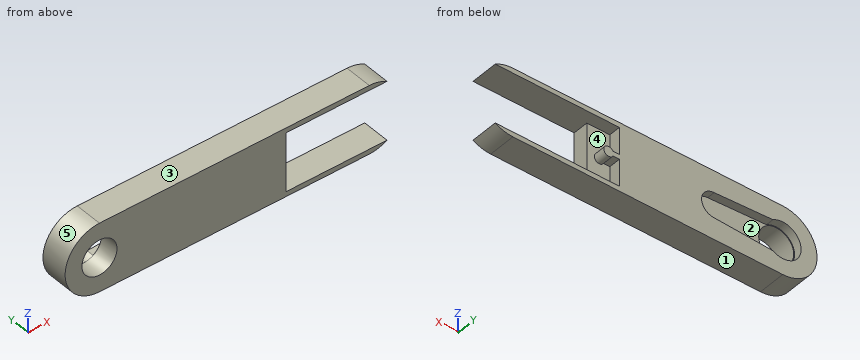
from build123d import *

# Parameters (mm, degrees)
BOSS_EXTRUDE1_DEPTH = 3.95
SKETCH2_R           = 3.575
CUT_EXTRUDE1_DEPTH  = 3.95
BOSS_EXTRUDE2_DEPTH = 1.64
SKETCH4_R           = 3.25
CUT_EXTRUDE2_DEPTH  = 63.643819328
CAVITY1_OUTLINE_R   = 3.25
CAVITY1_DEPTH       = 5.59
CAVITY1_START       = 3.19
CAVITY1_2_DEPTH     = 2.4
CUT_EXTRUDE4_DEPTH  = 63.643819328


# Read off the part's stored shape, not the designer's step: Cavity1
with BuildPart() as part:
    # Sketch1 → Boss-Extrude1 (new body)
    with BuildSketch(Plane(origin=(0, 0, 0), x_dir=(1, 0, 0), z_dir=(0, 1, 0))):
        with BuildLine():
            Line((0, 7), (55, 7))
            ThreePointArc((55, 7), (62, 0), (55, -7))
            Line((55, -7), (0, -7))
            ThreePointArc((0, -7), (-7, 0), (0, 7))
        make_face()
    extrude(amount=BOSS_EXTRUDE1_DEPTH)

    # Sketch2 → Cut-Extrude1 (cut)
    with BuildSketch(Plane.XZ):
        with Locations(Location((0, 0, 0), (0, 0, 270))):
            Circle(SKETCH2_R)
    extrude(amount=-CUT_EXTRUDE1_DEPTH, mode=Mode.SUBTRACT)

    # Sketch3 → Boss-Extrude2 (add)
    with BuildSketch(Plane(origin=(0, 3.95, 0), x_dir=(1, 0, 0), z_dir=(0, 1, 0))):
        with BuildLine():
            Line((0, -7), (55, -7))
            ThreePointArc((55, -7), (62, 0), (55, 7))
            Line((55, 7), (0, 7))
            ThreePointArc((0, 7), (-7, 0), (0, -7))
        make_face()
        with BuildLine():
            Line((13.979308982, 2.569996388), (1.997926282, 3.167540934))
            ThreePointArc((1.997926282, 3.167540934), (-3.745, 0), (1.997926282, -3.167540934))
            Line((1.997926282, -3.167540934), (13.979308982, -2.569996388))
            ThreePointArc((13.979308982, -2.569996388), (16.545, 0), (13.979308982, 2.569996388))
        make_face(mode=Mode.SUBTRACT)
    extrude(amount=BOSS_EXTRUDE2_DEPTH)

    # Sketch4 → Cut-Extrude2 (cut, through all)
    with BuildSketch(Plane(origin=(0, 5.59, 0), x_dir=(1, 0, 0), z_dir=(0, 1, 0))):
        with Locations(Location((55, 0, 0), (0, 0, 270))):
            Circle(SKETCH4_R)
    extrude(amount=-CUT_EXTRUDE2_DEPTH, mode=Mode.SUBTRACT)

    # Cavity1 outline → Cavity1 (cut)
    with BuildSketch(Plane(origin=(0, 0, 0), x_dir=(1, 0, 0), z_dir=(0, 1, 0))):
        with BuildLine():
            Line((58.605551275, 6), (38, 6))
            Line((38, 6), (38, -6))
            Line((38, -6), (58.605551275, -6))
            ThreePointArc((58.605551275, -6), (59.949747468, -4.949747468), (61, -3.605551275))
            Line((61, -3.605551275), (61, 3.605551275))
            ThreePointArc((61, 3.605551275), (59.949747468, 4.949747468), (58.605551275, 6))
        make_face()
        with Locations((55, 0)):
            Circle(CAVITY1_OUTLINE_R, mode=Mode.SUBTRACT)
    extrude(amount=CAVITY1_DEPTH, mode=Mode.SUBTRACT)

    # Cavity1 2 outline → Cavity1 2 (cut)
    with BuildSketch(Plane(origin=(0, 0, 0), x_dir=(1, 0, 0), z_dir=(0, 1, 0)).offset(CAVITY1_START)):
        with BuildLine():
            Line((33.3, 0.5), (34.605619966, 0.5))
            ThreePointArc((34.605619966, 0.5), (36.47164537, 0), (34.605619966, -0.5))
            Line((34.605619966, -0.5), (33.3, -0.5))
            Line((33.3, -0.5), (33.3, -6))
            Line((33.3, -6), (38, -6))
            Line((38, -6), (38, 6))
            Line((38, 6), (33.3, 6))
            Line((33.3, 6), (33.3, 0.5))
        make_face()
        with BuildLine():
            ThreePointArc((61, -3.605551275), (62, 0), (61, 3.605551275))
            Line((61, 3.605551275), (61, -3.605551275))
        make_face()
    extrude(amount=CAVITY1_2_DEPTH, mode=Mode.SUBTRACT)

    # Sketch5 → Cut-Extrude4 (cut, through all)
    with BuildSketch(Plane.XZ):
        with BuildLine():
            Line((61, 3.605551275), (61, -3.605551275))
            ThreePointArc((61, -3.605551275), (62, 0), (61, 3.605551275))
        make_face()
    extrude(amount=-CUT_EXTRUDE4_DEPTH, mode=Mode.SUBTRACT)


solid = part.part
The listing builds one solid part. Answer for the finished solid, in the listing's coordinates (mm). Face numbers are marked on the shaded views. A direction names the side the tool comes from. Give positions to 0.01 mm unless a question says otherwise; leave off trailing zeros. Loops run counter-clockwise (first coordinate to the right, second up) from the corner with the lowest first, then second, coordinate; pieces in that order, holes last. Notation, with made-up numbers: (9.5, 1.5) - (68.5, 1.5) arc R8 cw to (68.5, 8.5) - close; hole circle Ø3 at (13, 27.25). An arc over 180 degrees is marked (long way). Use one line per item in the form item = value.
1. Section C-C on y = 1.55 is taken. Give the vertices of the cut face in (x, z) (3 decimals).
Calculated:
outline = (0, -7) - (55, -7) arc R7 ccw to (58.606, -6) - (38, -6) - (38, 6) - (58.606, 6) arc R7 ccw to (55, 7) - (0, 7) arc R7 ccw to start; hole circle Ø7.15 at (0, 0)
2. Section B-B on x = 1 is taken. Give the vertices of the cut face in (y, z).
Calculated:
outline = (0, -7) - (5.59, -7) - (5.59, -3.61) - (3.95, -3.61) - (3.95, -3.43) - (0, -3.43) - close; (0, 3.43) - (3.95, 3.43) - (3.95, 3.61) - (5.59, 3.61) - (5.59, 7) - (0, 7) - close
3. Section A-A on y = 4.5 is taken. Give the vertices of the cut face in (x, z) (3 decimals), then the cut area to 3 significant figures.
Calculated:
outline = (0, -7) - (55, -7) arc R7 ccw to (58.606, -6) - (33.3, -6) - (33.3, -0.5) - (34.606, -0.5) arc R1 ccw (long way) to (34.606, 0.5) - (33.3, 0.5) - (33.3, 6) - (58.606, 6) arc R7 ccw to (55, 7) - (0, 7) arc R7 ccw to start; hole (1.998, -3.168) - (13.979, -2.57) arc R2.57 ccw to (13.979, 2.57) - (1.998, 3.168) arc R3.745 ccw (long way) to start
area = 480 mm^2
4. Given pin 1 Ø6.5 at (x, z) = (0, 0) entering from -Y; pin 2 Ø2.5 at (y, z) = (4, -2.5) entering from +X; pin 3 Ø0.7 at (y, z) = (4, 3.5) entering from +X; pin 4 Ø4 at (x, z) = (36.5, 3) entering from +Y, each flat-ended and moving along its own axis, determine where each tip first touches the part or whether it passes through.
Calculated:
pin_1 = through
pin_2 = 38
pin_3 = 33.3
pin_4 = 3.19
5. Which of the six approach directions +Z, -Z, +X, -X, +Y, -Y give full straight-line access (tool end or side, diameter ignored) to the marked faces 1 and 2?
Calculated:
face_1 = -Z, +X, -X, +Y, -Y
face_2 = +Y
6. Find the intervals of material crossed by line 1 along X through (y, z) = (5.1, 0) (3 decimals); line 2 along X through (y, z) = (1.6, 0) (3 decimals); line 3 along Y through (x, z) = (11.5, 0.5), in increasing order. Write a range as [from, to].
Calculated:
line_1 = [-7, -3.745], [16.545, 36.472]
line_2 = [-7, -3.575], [3.575, 38]
line_3 = [0, 3.95]
7. Section D-D on z = -5.25 is taken. Give the vertices of the cut face in (x, y).
Calculated:
outline = (-4.63, 0) - (38, 0) - (38, 3.19) - (33.3, 3.19) - (33.3, 5.59) - (-4.63, 5.59) - close
8. The mould has two halves that part along Z. Classify the marked faces 3, 4 and 5: pulls with the +Z half, pulls with the -Z half, needs draft (parallel to the pull), parting line crosses it, or undercut.
Calculated:
face_3 = pulls with the +Z half
face_4 = undercut
face_5 = parting line crosses it
